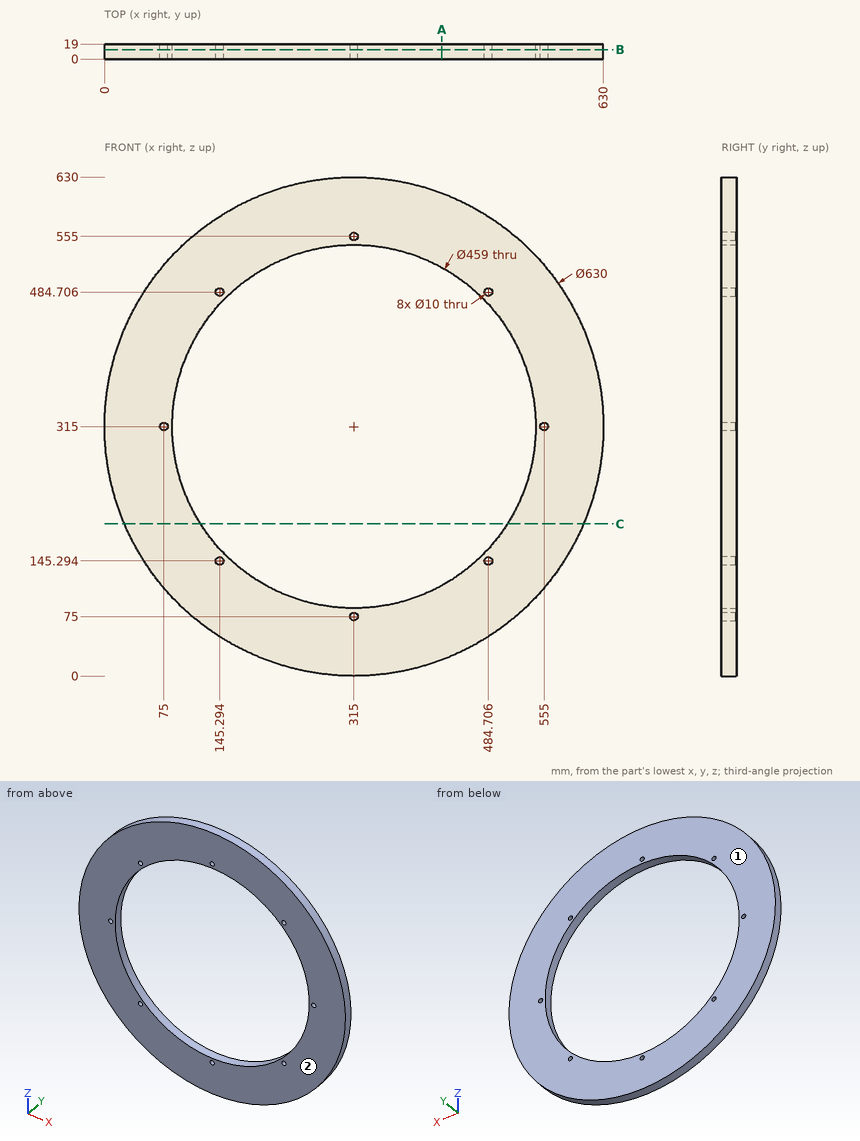
Study the drawing (mm; zero at the part's minimum x, y, z) and answer. Coordinates: 2 decimals unless noted, no trailing zeros. Order: outer loops, then holes, each group sorted by start corner. A loop starts at its lowest first (then second) coordinate and runs counter-clockwise, first axis right, second up. Notation, with made-up numbers: M 81.5,18.25 L 102.5,18.25 A11 cw 102.5,23.25 Z; hole C 66.5,7.25 d2. An arc over 180 degrees is marked long. Answer as a JSON object with one key per item and string values. Group by question number.
1. Section C-C on z = 192 is taken. Write down the section's boundary in (x, y) (1 decimal).
2. Straight lines are drawn through the part: line 1 (Z direction, x = 524, y = 2.5) (1 decimal); line 2 (Z direction, x = 231.5, y = 10.5); line 3 (X direction, y = 17, z = 416). For each, find the intervals that lie inside material, in ascending order.
3. Flat-ended cylindrical pins translate along their axes: P1, Ø5, axis at x = 359, y = 2.5, coming from the +Z side; P2, Ø6, axis at y = 3, z = 447.5, coming from the +X side; P3, Ø5, axis at y = 10, z = 112, coming from the -X side. Find the tip coordinate at first contact, or state that the pin passes through.
4. Section B-B on y = 12 is taken. State how many separate pieces and enclosed holes the cut face has, then the cut area to 3 significant figures.
5. Section A-A on x = 426 is taken. Write down the section's boundary in (y, z) (1 decimal).
6. Determine the mould class of the marked faces 1 and 2 for opening direction Y: released by +Y, released by -Y, zero draft, split by the parting line, or undercut.
Values follow:
{
 "1": {"outline": "M 25,0 L 121.2,0 L 121.2,19 L 25,19 Z; M 508.8,0 L 605,0 L 605,19 L 508.8,19 Z"},
 "2": {"line 1": "79.3 to 220.2, 409.8 to 550.7", "line 2": "11.27 to 101.23, 528.77 to 618.73", "line 3": "16.63 to 108.92, 521.08 to 613.37"},
 "3": {"P1": "z = 627.25", "P2": "x = 602.15", "P3": "x = 72.05"},
 "4": {"separate pieces": "1", "enclosed holes": "9", "area": "146,000 mm2"},
 "5": {"outline": "M 0,20.2 L 19,20.2 L 19,114.1 L 0,114.1 Z; M 0,515.9 L 19,515.9 L 19,609.8 L 0,609.8 Z"},
 "6": {"face 1": "released by +Y", "face 2": "released by -Y"}
}
